```python
from build123d import *

# Parameters (mm, degrees)
F0_W      = 170
F0_H      = 45
F1_DEPTH  = 52.5
F3_D      = 10
F5_DEPTH  = 45.001
F6_W      = 30
F6_H      = 37.5
F7_DEPTH  = 170.001
F9_D      = 10
F11_DEPTH = 45.001
F12_R     = 15
F14_DEPTH = 15
F16_DEPTH = 25


with BuildPart() as f1:
    # F0 (on Top) → F1 (new body)
    with BuildSketch(Plane.XY):
        Rectangle(F0_W, F0_H)
    extrude(amount=F1_DEPTH)

    # F3 (through all)
    with Locations(Plane.XY.offset(52.5)):
        with Locations((-65, 5.5), (65, 5.5)):
            Hole(F3_D / 2)

    # F4 (on face) → F5 (cut, through all)
    with BuildSketch(Plane.XZ.offset(22.5)):
        with BuildLine():
            Line((-85, 0), (85, 0))
            ThreePointArc((85, 0), (0, 27.5), (-85, 0))
        make_face()
    extrude(amount=-F5_DEPTH, mode=Mode.SUBTRACT)

    # F6 (on face) → F7 (cut, through all)
    with BuildSketch(Plane.YZ.offset(85)):
        with Locations((7.5, 18.75)):
            Rectangle(F6_W, F6_H)
    extrude(amount=-F7_DEPTH, mode=Mode.SUBTRACT)

    # F9 (through all)
    with Locations(Plane.XZ.offset(22.5)):
        with Locations((-75, 24.5), (75, 24.5)):
            Hole(F9_D / 2)

    # F10 (on face) → F11 (cut, through all)
    with BuildSketch(Plane.XZ.offset(22.5)):
        with BuildLine():
            ThreePointArc((85, 24.5), (81.246693, 16.691106), (72.804234, 14.744047))
            Line((72.804234, 14.744047), (31.863562, 23.958539))
            Line((31.863562, 23.958539), (85, 0))
            Line((85, 0), (85, 24.5))
        make_face()
        with BuildLine():
            ThreePointArc((-72.804234, 14.744047), (-81.246693, 16.691106), (-85, 24.5))
            Line((-85, 24.5), (-85, 0))
            Line((-85, 0), (-31.863562, 23.958539))
            Line((-31.863562, 23.958539), (-72.804234, 14.744047))
        make_face()
    extrude(amount=-F11_DEPTH, mode=Mode.SUBTRACT)

    # F12
    f12_edges = [f1.edges().sort_by_distance(p)[0] for p in [
        (85, 22.5, 45),
        (-85, 22.5, 45),
    ]]
    fillet(f12_edges, radius=F12_R)

    # F13 (on face) → F14 (join, through all)
    with BuildSketch(Plane.XZ.offset(22.5)):
        Polygon((-48.969162, 34.744047), (-72.804234, 14.744047), (72.804234, 14.744047), (48.969162, 34.744047), align=None)
    extrude(amount=-F14_DEPTH)

    # F15 (on face) → F16 (cut)
    with BuildSketch(Plane.XZ.offset(22.5)):
        Polygon((-15, 27.744047), (-72.804234, 14.744047), (72.804234, 14.744047), (15, 27.744047), align=None)
    extrude(amount=-F16_DEPTH, mode=Mode.SUBTRACT)


solid = f1.part
```
CAD build for the part. Positions are in the model's coordinates, mm. A direction names the side the tool comes from. Round coordinates to 2 decimals unless told otherwise and drop trailing zeros. Write each loop counter-clockwise with the first axis right and the second up, starting at its lowest first coordinate (ties: lowest second). Pieces come first, ordered by that corner, then holes. Notation, with made-up numbers: (10, 30.25) - (20, 30.25) arc R9 cw to (20, 39.25) - close; hole circle Ø11 at (83.5, 53.25). An arc over 180 degrees is marked (long way). Write item = value, one per line. Start each with the question number.
Q1. Which spindle directions (+Z, -Z, +X, -X, +Y, -Y) get a long thin tool onto all of the face, cutting with end or side? Do faces 5 (the flat face through (44.307, -15.105, 21.153)), 6 (the flat face through (1, -7.5, 28)), 7 (the cylindrical face through (69.995, 5.72, 44.895)). Say none if no direction does.
Q2. Band-saw the part on A-A (z = 50.5). Give the cut face in (x, y).
Q3. Drop flat-ended pins along their axis: pin 1 (9 mm diameter, centred on x = 65, y = 5.5, fed in from +Z); pin 2 (24 mm diameter, centred on x = 1, y = 7.5, fed in from -Z); pin 3 (1 mm diameter, centred on x = -60.5, z = 21.5, fed in from +Y); pin 4 (6 mm diameter, centred on y = 14, z = 48, fed in from +X). Give the stop position or say it passes through.
Q4. Mould opens along X. For faces 1 (the cylindrical face through (-63.92, 0.62, 44.9)), 2 (the flat face through (0, -15, 27.744)), 3 (the flat face through (-1, 0, 52.5)), 4 (the cylindrical face through (80.49, 18.22, 45.1)) say: pulls with the +X half, pulls with the -X half, needs draft (parallel to the pull), parting line crosses it, or undercut.
Q5. Band-saw the part on B-B (y = -19). Give the cut face in (x, z), then the cut area to 3 significant figures.
Q6. Band-saw the part on D-D (x = -13). Give the cut face in (y, z).
Q7. Band-saw the part on C-C (x = -65). Give the cut face in (y, z).
Q8. Probe L1, parallel to Y at x = 46, z = 37; L2, parallel to Y at x = -65, z = 49; L3, parallel to Z at x = 75, y = -13.75. List the from-to ranges inside material, lowest first. Write a range as from..to.
Answers below:
q1.face_5 = -Z, +Y, -Y
q1.face_6 = -Z, +X, -X, +Y
q1.face_7 = +Z, -Z
q2.outline = (-85, -22.5) - (85, -22.5) - (85, 7.5) arc R15 ccw to (70, 22.5) - (-70, 22.5) arc R15 ccw to (-85, 7.5) - close; hole circle Ø10 at (-65, 5.5); hole circle Ø10 at (65, 5.5)
q3.pin_1 = through
q3.pin_2 = 37.5
q3.pin_3 = -7.5
q3.pin_4 = 84.59
q4.face_1 = undercut
q4.face_2 = undercut
q4.face_3 = needs draft
q4.face_4 = pulls with the +X half
q5.outline = (-85, 24.5) arc R10 ccw to (-72.8, 14.74) - (-15, 27.74) - (15, 27.74) - (72.8, 14.74) arc R10 ccw to (85, 24.5) - (85, 52.5) - (-85, 52.5) - close; hole circle Ø10 at (-75, 24.5); hole circle Ø10 at (75, 24.5)
q5.area = 5,080 mm2
q6.outline = (-22.5, 27.74) - (-7.5, 27.74) - (-7.5, 37.5) - (22.5, 37.5) - (22.5, 52.5) - (-22.5, 52.5) - close
q7.outline = (-22.5, 16.5) - (-7.5, 16.5) - (-7.5, 37.5) - (0.5, 37.5) - (0.5, 52.5) - (-22.5, 52.5) - close; (10.5, 37.5) - (22.5, 37.5) - (22.5, 52.5) - (10.5, 52.5) - close
q8.L1 = -22.5..-7.5
q8.L2 = -22.5..0.5, 10.5..22.5
q8.L3 = 14.5..19.5, 29.5..52.5
